Geometry check sheet. Reference: the model listing, model coordinates, mm. Face numbers are marked on the shaded views. A direction names the side the tool comes from. Round coordinates to 2 decimals unless told otherwise and drop trailing zeros. Order: outer loops, then holes, each group sorted by start corner. A loop starts at its lowest first (then second) coordinate and runs counter-clockwise, first axis right, second up. Notation, with made-up numbers: (63, -28.75) - (109, -28.75) arc R36 ccw to (109, 7.25) - close; hole circle Ø6 at (1, -16). An arc over 180 degrees is marked (long way). Answer as CSV lines item,"result". Start each with the question number.
```python
from build123d import *

# Parameters (mm, degrees)
F1_DEPTH = 7.5
F2_DEPTH = 3
F3_DEPTH = 6.5
F4_W     = 5.6182215922
F4_H     = 5.2901296224
F4_W_2   = 4.8481553793
F4_H_2   = 2.1686895564
F4_W_3   = 11.6345733404
F4_H_3   = 1.9571522065
F4_W_4   = 3.1425692141
F4_W_5   = 9.7834728658
F4_W_6   = 16.2676852196
F4_W_7   = 3.9411410689
F4_W_8   = 3.3481553793
F5_DEPTH = 2
F6_R     = 1


with BuildPart() as f1:
    # F0 (on Front) → F1 (new body)
    with BuildSketch(Plane.XZ):
        Polygon((-48.5, 2), (-48.5, 0), (50, 0), (50, 2), (40.15, 2), (16.9, 2), (12.75, 2), (0.75, 2), (-11.25, 2), (-15.4, 2), (-38.65, 2), align=None)
    extrude(amount=F1_DEPTH)

    # F0 (on Front) → F2 (join)
    with BuildSketch(Plane.XZ):
        with BuildLine():
            Line((16.9, 2), (40.15, 2))
            Line((40.15, 2), (35.9, 11))
            ThreePointArc((35.9, 11), (28.9, 4), (21.9, 11))
            Line((21.9, 11), (16.9, 2))
        make_face()
        with BuildLine():
            Line((0.75, 2), (12.75, 2))
            Line((12.75, 2), (7.75, 11))
            ThreePointArc((7.75, 11), (5.6997474683, 6.0502525317), (0.75, 4))
            Line((0.75, 4), (0.75, 2))
        make_face()
        with BuildLine():
            Line((-6.25, 11), (-11.25, 2))
            Line((-11.25, 2), (0.75, 2))
            Line((0.75, 2), (0.75, 4))
            ThreePointArc((0.75, 4), (-4.1997474683, 6.0502525317), (-6.25, 11))
        make_face()
        with BuildLine():
            Line((-34.4, 11), (-38.65, 2))
            Line((-38.65, 2), (-15.4, 2))
            Line((-15.4, 2), (-20.4, 11))
            ThreePointArc((-20.4, 11), (-27.4, 4), (-34.4, 11))
        make_face()
        Polygon((-48.5, 2), (-48.5, 0), (50, 0), (50, 2), (40.15, 2), (16.9, 2), (12.75, 2), (0.75, 2), (-11.25, 2), (-15.4, 2), (-38.65, 2), align=None)
    extrude(amount=-F2_DEPTH)

    # F0 (on Front) → F3 (join)
    with BuildSketch(Plane.XZ):
        Polygon((-48.5, 2), (-48.5, 0), (50, 0), (50, 2), (40.15, 2), (16.9, 2), (12.75, 2), (0.75, 2), (-11.25, 2), (-15.4, 2), (-38.65, 2), align=None)
    extrude(amount=-F3_DEPTH)

    # F4 (on face) → F5 (cut)
    with BuildSketch(Plane.XY.offset(2)):
        with Locations((6.8839930464, -4.8549351888)):
            Rectangle(F4_W, F4_H)
        with Locations((47.5759223104, 5.4156552218)):
            Rectangle(F4_W_2, F4_H_2)
        with Locations((27.9820300639, 5.5214238968)):
            Rectangle(F4_W_3, F4_H_3)
        with Locations((39.5776275545, 5.5214238968)):
            Rectangle(F4_W_4, F4_H_3)
        with Locations((9.5749795437, 5.5214238968)):
            Rectangle(F4_W_5, F4_H_3)
        with Locations((28.3925579861, -4.8549351888)):
            Rectangle(F4_W_6, F4_H)
        with Locations((43.8636317849, -4.8549351888)):
            Rectangle(F4_W_7, F4_H)
        with Locations((-6.8839930464, -4.8549351888)):
            Rectangle(F4_W, F4_H)
        with Locations((-9.5749795437, 5.5214238968)):
            Rectangle(F4_W_5, F4_H_3)
        with Locations((-28.3925579861, -4.8549351888)):
            Rectangle(F4_W_6, F4_H)
        with Locations((-27.9820300639, 5.5214238968)):
            Rectangle(F4_W_3, F4_H_3)
        with Locations((-39.5776275545, 5.5214238968)):
            Rectangle(F4_W_4, F4_H_3)
        with Locations((-43.8636317849, -4.8549351888)):
            Rectangle(F4_W_7, F4_H)
        with Locations((-46.8259223104, 5.4156552218)):
            Rectangle(F4_W_8, F4_H_2)
    extrude(amount=-F5_DEPTH, mode=Mode.SUBTRACT)

    # F6
    f6_edges = [f1.edges().sort_by_distance(p)[0] for p in [
        (35.9, 1.5, 11),
        (21.9, 1.5, 11),
        (7.75, 1.5, 11),
        (-6.25, 1.5, 11),
        (-20.4, 1.5, 11),
        (-34.4, 1.5, 11),
    ]]
    fillet(f6_edges, radius=F6_R)


solid = f1.part
```
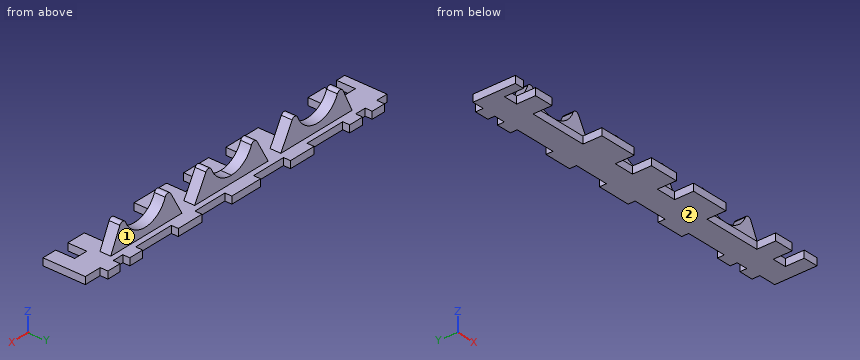
1. Section check D-D on x = 24. Record the boundary of the cut face in (y, z).
2. Go/stop test with flat-tipped pins: pin 1 Ø0.6 at (y, z) = (5.5, 1) entering from +X; pin 2 Ø2 at (y, z) = (2, 3.5) entering from +X; pin 3 Ø2 at (y, z) = (5.5, 0.5) entering from -X. Record where each tip stops, or that it passes through.
3. Section check C-C on y = 1. Record the boundary of the cut face in (x, z), plus the area to 3 significant figures.
4. Section check B-B on z = 7. Record the boundary of the cut face in (x, y), plus the area to 3 significant figures.
5. Access from +Z, -Z, +X, -X, +Y, -Y to the whole of each face (thin tool, end or side, straight path). Record for the marked faces 1 and 2.
6. Thickness scan on probe 1 along X at (y, z) = (2, 3.5); probe 2 along X at (y, z) = (1, 8); probe 3 along X at (y, z) = (1, 2.25). Record the ranges inside material, lowest first.
7. Section check A-A on y = -3.25. Record the boundary of the cut face in (x, z).
Numbers:
1,outline,"(-2.21, 0) - (4.54, 0) - (4.54, 2) - (3, 2) - (3, 6) - (0, 6) - (0, 2) - (-2.21, 2) - close"
2,pin 1,"stops at x = 45.15"
2,pin 2,"stops at x = 39.91"
2,pin 3,"stops at x = -45.15"
3,outline,"(-48.5, 0) - (50, 0) - (50, 2) - (40.15, 2) - (37.17, 8.31) arc R1 ccw to (35.35, 8.27) arc R7 cw to (22.37, 8.47) arc R1 ccw to (20.57, 8.6) - (16.9, 2) - (12.75, 2) - (9.08, 8.6) arc R1 ccw to (7.28, 8.47) arc R7 cw to (-5.78, 8.47) arc R1 ccw to (-7.58, 8.6) - (-11.25, 2) - (-15.4, 2) - (-19.07, 8.6) arc R1 ccw to (-20.87, 8.47) arc R7 cw to (-33.85, 8.27) arc R1 ccw to (-35.67, 8.31) - (-38.65, 2) - (-48.5, 2) - close"
3,area,"464 mm2"
4,outline,"(-36.29, 0) - (-33.14, 0) - (-33.14, 3) - (-36.29, 3) - close; (-21.66, 0) - (-18.18, 0) - (-18.18, 3) - (-21.66, 3) - close; (-8.47, 0) - (-4.99, 0) - (-4.99, 3) - (-8.47, 3) - close; (6.49, 0) - (9.97, 0) - (9.97, 3) - (6.49, 3) - close; (19.68, 0) - (23.16, 0) - (23.16, 3) - (19.68, 3) - close; (34.64, 0) - (37.79, 0) - (37.79, 3) - (34.64, 3) - close"
4,area,"60.6 mm2"
5,face 1,"+Z, +X, -X, +Y"
5,face 2,"-Z, +X, -X, +Y, -Y"
6,probe 1,"x = -37.94 to -16.23, -10.42 to 11.92, 17.73 to 39.44"
6,probe 2,"x = -35.82 to -33.72, -21.08 to -18.73, -7.92 to -5.57, 7.07 to 9.42, 20.23 to 22.58, 35.22 to 37.32"
6,probe 3,"x = -38.53 to -15.54, -11.11 to 12.61, 17.04 to 40.03"
7,outline,"(-48.5, 0) - (-45.83, 0) - (-45.83, 2) - (-48.5, 2) - close; (-41.89, 0) - (-36.53, 0) - (-36.53, 2) - (-41.89, 2) - close; (-20.26, 0) - (-9.69, 0) - (-9.69, 2) - (-20.26, 2) - close; (-4.07, 0) - (4.07, 0) - (4.07, 2) - (-4.07, 2) - close; (9.69, 0) - (20.26, 0) - (20.26, 2) - (9.69, 2) - close; (36.53, 0) - (41.89, 0) - (41.89, 2) - (36.53, 2) - close; (45.83, 0) - (50, 0) - (50, 2) - (45.83, 2) - close"
